Check sheet for the modelled part. Datum: model origin and axes. Units: mm. A direction names the side the tool comes from. Round coordinates to 2 decimals unless told otherwise and drop trailing zeros. Loops run counter-clockwise (first coordinate to the right, second up) from the corner with the lowest first, then second, coordinate; pieces in that order, holes last. Notation, with made-up numbers: (31, 85.25) - (60, 85.25) arc R27 ccw to (60, 119.25) - close; hole circle Ø4 at (-31.5, 36). An arc over 180 degrees is marked (long way). Put each result on its own line as item: value. Start each with the question number.
Item 1: Material ranges on line 1 along Z through (x, y) = (-12.5, 1.4); line 2 along X through (y, z) = (0.35, -1.75); line 3 along X through (y, z) = (1.8, 2.5), recorded low to high.
Item 2: Tool access check on faces 1 (the flat face through (-8, 2, 0)), 2 (the flat face through (-9, 1, 3.81)), 3 (the flat face through (-0.1, 0.5, 6)), 4 (the flat face through (-1, 0, 0)), 5 (the flat face through (-9, 1, -3.81)). Record the directions out of +Z, -Z, +X, -X, +Y, -Y that give a thin tool (end or side, any length) a straight path to the whole face; none if there is none.
Item 3: Gauge pin test, flat ends, axial feed: pin 1 Ø0.5 at (x, z) = (-14.5, 2.5) entering from -Y; pin 2 Ø0.8 at (y, z) = (0.5, 4.5) entering from -X; pin 3 Ø3 at (x, z) = (3, 1) entering from +Y. Record the tip position at first contact, or that the pin passes through.
Item 4: Section check A-A, the plane x = -11.5. Record the cut outline in (y, z).
Item 5: Section check B-B, the plane y = 0.5. Record the cut outline in (x, z), and give its area (3 significant figures).
Item 6: Section check D-D, the plane x = -5. Record the cut outline in (y, z), and give its area (3 significant figures).
Item 7: Section check C-C, the plane z = 1. Record the cut outline in (x, y).
from build123d import *

# Parameters (mm, degrees)
BOSS_EXTRU_1_DEPTH = 1
ESQUISSE2_W        = 2.54
ESQUISSE2_H        = 2.54
BOSS_EXTRU_2_DEPTH = 3.81
ESQUISSE3_W        = 0.6
ESQUISSE3_H        = 0.6
BOSS_EXTRU_3_DEPTH = 6
CHANFREIN1_SIZE    = 0.2


with BuildPart() as part:
    # Esquisse1 → Boss.-Extru.1 (new body)
    with BuildSketch(Plane(origin=(0, 0, 0), x_dir=(1, 0, 0), z_dir=(0, 1, 0))):
        with BuildLine():
            Line((-6.5, -6), (6.5, -6))
            ThreePointArc((6.5, -6), (6.939339828, -4.939339828), (8, -4.5))
            Line((8, -4.5), (8, 4.5))
            ThreePointArc((8, 4.5), (6.939339828, 4.939339828), (6.5, 6))
            Line((6.5, 6), (-6.5, 6))
            ThreePointArc((-6.5, 6), (-6.939339828, 4.939339828), (-8, 4.5))
            Line((-8, 4.5), (-8, -4.5))
            ThreePointArc((-8, -4.5), (-6.939339828, -4.939339828), (-6.5, -6))
        make_face()
    extrude(amount=BOSS_EXTRU_1_DEPTH)

    # Esquisse2 → Boss.-Extru.2 (add, symmetric)
    with BuildSketch(Plane(origin=(0, 0, 0), x_dir=(-1, 0, 0), z_dir=(0, 0, -1))):
        with Locations((9.27, 1.27)):
            Rectangle(ESQUISSE2_W, ESQUISSE2_H)
    extrude(amount=BOSS_EXTRU_2_DEPTH, both=True)

    # Esquisse3 → Boss.-Extru.3 (add)
    with BuildSketch(Plane.ZY.offset(10.54)):
        with Locations((-2.54, 1.27)):
            Rectangle(ESQUISSE3_W, ESQUISSE3_H)
        with Locations((0, 1.27)):
            Rectangle(ESQUISSE3_W, ESQUISSE3_H)
        with Locations((2.54, 1.27)):
            Rectangle(ESQUISSE3_W, ESQUISSE3_H)
    extrude(amount=BOSS_EXTRU_3_DEPTH)

    # Chanfrein1
    chanfrein1_edges = [part.edges().sort_by_distance(p)[0] for p in [
        (-16.54, 1.27, -2.84),
        (-16.54, 0.97, -2.54),
        (-16.54, 1.27, -2.24),
        (-16.54, 1.57, -2.54),
        (-16.54, 1.27, -0.3),
        (-16.54, 0.97, 0),
        (-16.54, 1.27, 0.3),
        (-16.54, 1.57, 0),
        (-16.54, 1.27, 2.24),
        (-16.54, 0.97, 2.54),
        (-16.54, 1.27, 2.84),
        (-16.54, 1.57, 2.54),
    ]]
    chamfer(chanfrein1_edges, length=CHANFREIN1_SIZE)


solid = part.part
Check result:
1. line 1: -2.84 to -2.24, -0.3 to 0.3, 2.24 to 2.84
1. line 2: -10.54 to 8
1. line 3: -10.54 to -8
2. face 1: +Z, -Z, +X, +Y
2. face 2: +Z, -X, +Y, -Y
2. face 3: +Z, +X, -X, +Y, -Y
2. face 4: +Z, -Z, +X, -X, -Y
2. face 5: -Z, -X, +Y, -Y
3. pin 1: y = 0.97
3. pin 2: x = -8
3. pin 3: y = 1
4. outline: (0.97, -2.84) - (1.57, -2.84) - (1.57, -2.24) - (0.97, -2.24) - close; (0.97, -0.3) - (1.57, -0.3) - (1.57, 0.3) - (0.97, 0.3) - close; (0.97, 2.24) - (1.57, 2.24) - (1.57, 2.84) - (0.97, 2.84) - close
5. outline: (-10.54, -3.81) - (-8, -3.81) - (-8, -4.5) arc R1.5 cw to (-6.5, -6) - (6.5, -6) arc R1.5 cw to (8, -4.5) - (8, 4.5) arc R1.5 cw to (6.5, 6) - (-6.5, 6) arc R1.5 cw to (-8, 4.5) - (-8, 3.81) - (-10.54, 3.81) - close
5. area: 204 mm²
6. outline: (0, -6) - (1, -6) - (1, 6) - (0, 6) - close
6. area: 12.0 mm²
7. outline: (-10.54, 0) - (8, 0) - (8, 1) - (-8, 1) - (-8, 2.54) - (-10.54, 2.54) - close
